Work out the finished part from the listing and answer in its coordinate system (mm). A direction names the side the tool comes from. Round coordinates to 2 decimals unless told otherwise and drop trailing zeros. Order: outer loops, then holes, each group sorted by start corner. A loop starts at its lowest first (then second) coordinate and runs counter-clockwise, first axis right, second up. Notation, with made-up numbers: (44.25, 18) -> (76.25, 18) arc R10 ccw to (76.25, 26) -> close; hole circle Ø2 at (-3.75, 2). An arc over 180 degrees is marked (long way). Use a Markdown table: item, result. Add a question column.
Item 1: A tool of negligible diameter and unlimited length cuts with its end or side. For faces 1 (the flat face through (10.79, -51.06, 77.94)), 2 (the flat face through (0, -13.74, 80)), 3 (the flat face through (-29, -21.064, 62)), 4 (the flat face through (32, -5, 0)), 5 (the flat face through (10.49, -51.06, 41.09)), from which of +Z, -Z, +X, -X, +Y, -Y can it reach the whole face along a straight path? Write none if from no direction.
Item 2: A cutting plane is placed at C-C, the plane y = -42. Determine the outline of the cut face in (x, z), plus the area to 3 significant figures.
Item 3: A cutting plane is placed at D-D, the plane x = 14. Determine the outline of the cut face in (y, z).
Item 4: For a pull along Y with two mould halves and no side action, classify faces 6 (the flat face through (-10.787, -21.237, 41.263)), 7 (the flat face through (-31, -2, 80.983)), 8 (the flat face through (-21.275, -51, 60)), 9 (the flat face through (22, -38.74, 49)) as +Y half, -Y half, draft (parallel to the pull), parting line (faces both ways), or undercut.
Item 5: A cutting plane is placed at A-A, the plane z = 62.5. Determine the outline of the cut face in (x, y), plus the area to 3 significant figures.
Item 6: Flat-ended cylindrical pins translate along their axes: P1, Ø12, axis at y = -52.5, z = 88, coming from the +X side; P2, Ø3, axis at x = -17, y = -42.5, coming from the +Z side; P3, Ø10, axis at x = 10, y = -22.5, coming from the -Z side. Find the tip coordinate at first contact, or state that the pin passes through.
Item 7: Find the intervals of material crossed by L1, parallel to X at y = -5.5, z = 95; L2, parallel to X at y = -22, z = 56; L3, parallel to X at y = 10.5, z = 37.5, in increasing order. Write a range as [from, to].
Item 8: A cutting plane is placed at B-B, the plane x = 35. Determine the outline of the cut face in (y, z).
from build123d import *

# Parameters (mm, degrees)
F0_W          = 67.3185419291
F0_H          = 69.4296189758
F1_DEPTH      = 100
F2_R          = 28.4134065768
F3_DEPTH      = 100.001
F5_DEPTH      = 25
F5_DEPTH_BACK = 25
F6_DEPTH      = 25
F8_DEPTH      = 92.3195419291


with BuildPart() as f1:
    # F0 (on Top) → F1 (new body)
    with BuildSketch(Plane.XY):
        with Locations((-0.362903811, -4.0251101746)):
            Rectangle(F0_W, F0_H)
    extrude(amount=F1_DEPTH)

    # F2 (on face) → F3 (cut, through all)
    with BuildSketch(Plane.XY.offset(100)):
        with Locations((0, -4.2641130276)):
            Circle(F2_R)
    extrude(amount=-F3_DEPTH, mode=Mode.SUBTRACT)

    # F4 (on face) → F5 (join, two sides)
    with BuildSketch(Plane.XZ.offset(38.7399196625)) as f5_sk:
        Polygon((-21.2752018124, 71.8850533229), (-21.2752018124, 47.318566336), (0, 35.0353228426), (21.2752018124, 47.318566336), (21.2752018124, 71.8850533229), (0, 84.1682968164), align=None)
    extrude(amount=F5_DEPTH)
    extrude(f5_sk.sketch, amount=-F5_DEPTH_BACK)

    # F6 (add): a face of the model
    f6_faces = [f1.faces().sort_by_distance(p)[0] for p in [
        (33.2963671535, -4.0251101746, 50),
    ]]
    extrude(f6_faces, amount=F6_DEPTH)

    # F7 (on face) → F8 (cut, through all)
    with BuildSketch(Plane(origin=(-34.0221747756, 0, 0), x_dir=(0, -1, 0), z_dir=(-1, 0, 0))):
        Polygon((21.0635084659, 54.3380566401), (21.0635084659, 69.9462256865), (10.0268662913, 80.9828678612), (-5.5813027551, 80.9828678612), (-16.6179449297, 69.9462256865), (-16.6179449297, 54.3380566401), (-5.5813027551, 43.3014144655), (10.0268662913, 43.3014144655), align=None)
    extrude(amount=-F8_DEPTH, mode=Mode.SUBTRACT)


solid = f1.part
Reported:
| question | item | result |
|---|---|---|
| 1 | face 1 | +Z, +X, -Y |
| 1 | face 2 | +Z, -Z |
| 1 | face 3 | +X, -X |
| 1 | face 4 | -Z, +X, -X, +Y, -Y |
| 1 | face 5 | -Z, +X, -Y |
| 2 | outline | (-21.28, 47.32) -> (0, 35.04) -> (21.28, 47.32) -> (21.28, 71.89) -> (0, 84.17) -> (-21.28, 71.89) -> close |
| 2 | area | 1,570 mm² |
| 3 | outline | (-63.74, 43.12) -> (-38.74, 43.12) -> (-38.74, 0) -> (-28.99, 0) -> (-28.99, 43.12) -> (-13.74, 43.12) -> (-13.74, 47.01) -> (-21.06, 54.34) -> (-21.06, 69.95) -> (-14.92, 76.09) -> (-28.99, 76.09) -> (-28.99, 100) -> (-38.74, 100) -> (-38.74, 76.09) -> (-63.74, 76.09) -> close; (20.46, 0) -> (30.69, 0) -> (30.69, 100) -> (20.46, 100) -> close |
| 4 | face 6 | undercut |
| 4 | face 7 | undercut |
| 4 | face 8 | draft |
| 4 | face 9 | -Y half |
| 5 | outline | (-34.02, -38.74) -> (-21.28, -38.74) -> (-21.28, -63.74) -> (21.28, -63.74) -> (21.28, -38.74) -> (58.3, -38.74) -> (58.3, -21.06) -> (22.92, -21.06) arc R28.41 cw to (21.28, -23.1) -> (21.28, -21.06) -> (-21.28, -21.06) -> (-21.28, -23.1) arc R28.41 cw to (-22.92, -21.06) -> (-34.02, -21.06) -> close; (-34.02, 16.62) -> (-19.27, 16.62) arc R28.41 cw to (19.27, 16.62) -> (58.3, 16.62) -> (58.3, 30.69) -> (-34.02, 30.69) -> close |
| 5 | area | 3,790 mm² |
| 6 | P1 | x = 3.76 |
| 6 | P2 | z = 75.22 |
| 6 | P3 | z = 37.92 |
| 7 | L1 | [-34.02, -28.39], [28.39, 58.3] |
| 7 | L2 | [-34.02, -22.2], [-21.28, 21.28], [22.2, 58.3] |
| 7 | L3 | [-34.02, -24.28], [24.28, 58.3] |
| 8 | outline | (-38.74, 0) -> (30.69, 0) -> (30.69, 100) -> (-38.74, 100) -> close; hole (-21.06, 54.34) -> (-10.03, 43.3) -> (5.58, 43.3) -> (16.62, 54.34) -> (16.62, 69.95) -> (5.58, 80.98) -> (-10.03, 80.98) -> (-21.06, 69.95) -> close |
